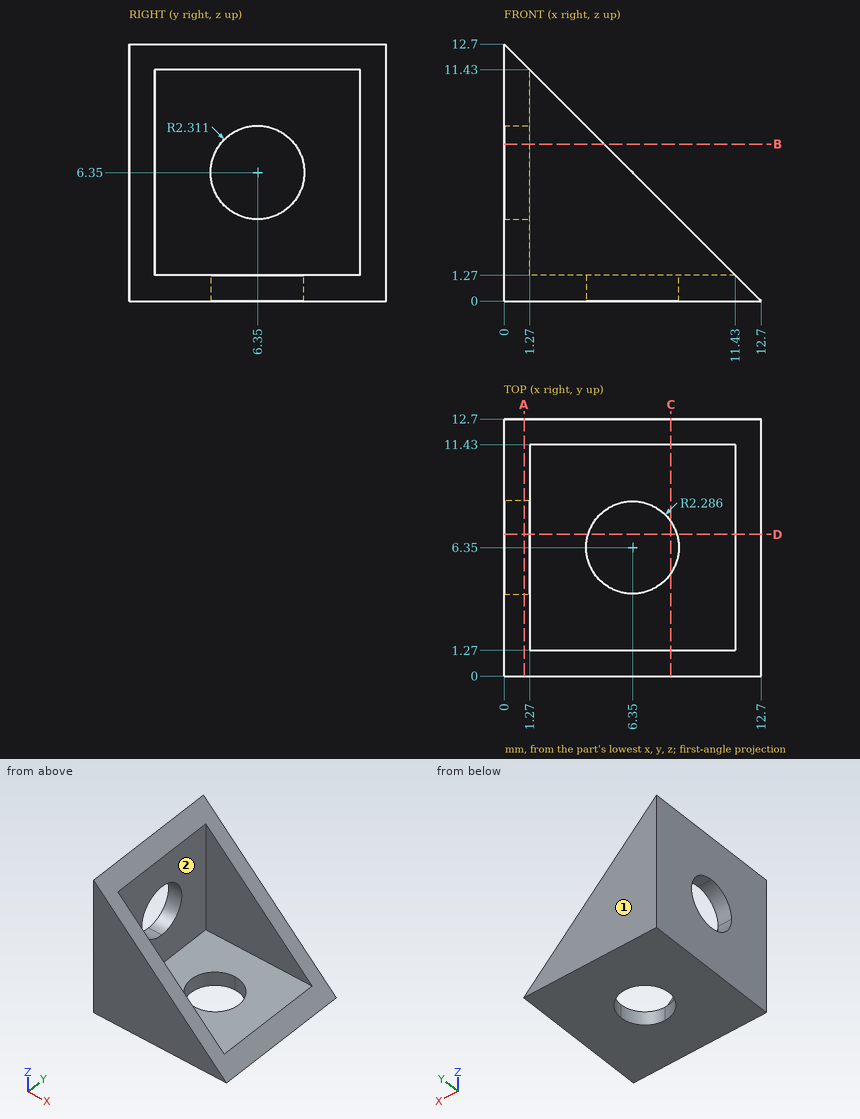
Part print with two shaded views. Sizes in mm from the minimum x, y, z corner. A direction names the side the tool comes from. Coordinates: 2 decimals unless noted, no trailing zeros. Write each loop counter-clockwise with the first axis right and the second up, starting at its lowest first coordinate (ties: lowest second). Pieces come first, ordered by that corner, then holes. Notation, with made-up numbers: (63, 43) -> (96, 43) arc R14 cw to (96, 55) -> close; hole circle Ø9 at (7.25, 81.25). An arc over 180 degrees is marked (long way). Return JSON: item names as keys, results as strings. Group by question number.
Q1. Cut at C-C, the plane x = 8.25. Give the cut face in (y, z).
Q2. Cut at A-A, the plane x = 1. Give the cut face in (y, z).
Q3. Flat gauge pins, fed straight in: pin 1 (5 mm diameter, centred on x = 7.5, y = 8, fed in from +Z); pin 2 (5 mm diameter, centred on y = 5.5, z = 6, fed in from +X); pin 3 (1 mm diameter, centred on y = 5, z = 6, fed in from -X). Where does each tip first touch, or does it go through?
Q4. Cut at D-D, the plane y = 7. Give the cut face in (x, z).
Q5. Cut at B-B, the plane z = 7.75. Give the cut face in (x, y), then the cut area to 3 significant figures.
Q6. Drill centre lines: line 1 (Y direction, x = 2.75, z = 2.75); line 2 (X direction, y = 11.25, z = 9). Where is each one in solid material? Low to high.
Q7. Which spindle directions (+Z, -Z, +X, -X, +Y, -Y) get a long thin tool onto all of the face, cutting with end or side? Do the marked faces 1 and 2. Say none if no direction does.
Returned:
{
 "1": {"outline": "(0, 0) -> (5.08, 0) -> (5.08, 1.27) -> (1.27, 1.27) -> (1.27, 4.45) -> (0, 4.45) -> close; (7.62, 0) -> (12.7, 0) -> (12.7, 4.45) -> (11.43, 4.45) -> (11.43, 1.27) -> (7.62, 1.27) -> close"},
 "2": {"outline": "(0, 0) -> (12.7, 0) -> (12.7, 11.7) -> (0, 11.7) -> close; hole circle Ø4.62 at (6.35, 6.35)"},
 "3": {"pin 1": "stops at z = 1.27", "pin 2": "stops at x = 1.27", "pin 3": "passes through"},
 "4": {"outline": "(0, 0) -> (4.16, 0) -> (4.16, 1.27) -> (1.27, 1.27) -> (1.27, 4.13) -> (0, 4.13) -> close; (0, 8.57) -> (1.27, 8.57) -> (1.27, 11.43) -> (0, 12.7) -> close; (8.54, 0) -> (12.7, 0) -> (11.43, 1.27) -> (8.54, 1.27) -> close"},
 "5": {"outline": "(0, 0) -> (4.95, 0) -> (4.95, 1.27) -> (1.27, 1.27) -> (1.27, 4.51) -> (0, 4.51) -> close; (0, 8.19) -> (1.27, 8.19) -> (1.27, 11.43) -> (4.95, 11.43) -> (4.95, 12.7) -> (0, 12.7) -> close", "area": "20.8 mm2"},
 "6": {"line 1": "y = 0 to 1.27, 11.43 to 12.7", "line 2": "x = 0 to 1.27"},
 "7": {"face 1": "+Z, -Z, +X, -X, +Y", "face 2": "+Z, +X"}
}
